Can you work these out from the model? Positions are in its coordinate system, mm. A direction names the side the tool comes from. Coordinates: 2 decimals unless noted, no trailing zeros. Return JSON: item names as keys, results as strings. Group by question number.
1) If we mould it in two halves opening along X, with no side actions, what happens to faces 1 (the face through (0, 0, 85)), 2 (the face through (-14.985, 0.66, 18.759)), 3 (the face through (-3, -10, 0)), 4 (the face through (-4.336, -19.524, 104.86))? For each: pulls with the +X half, pulls with the -X half, needs draft (parallel to the pull), parting line crosses it, or undercut.
2) If I drill on line 1 along Y through (x, z) = (0, 34.5); line 2 along Z through (x, y) = (11.5, 0); line 3 along Y through (x, z) = (0, 6), over which ranges is the centre line in solid material (lowest first)?
3) Which directions (+Z, -Z, +X, -X, +Y, -Y) give clear straight access to the entire face, cutting with the end or side of a thin tool? Please do faces 5 (the face through (0, 0, 95)), 6 (the face through (14.3, -14.3, 115)), 7 (the face through (0, 8.2, 13.797)).
4) For pin 1 Ø12 at (x, y) = (1.5, 4) entering from +Z; pin 2 Ø8 at (y, z) = (14, 68.5) entering from -X; pin 3 Ø0.7 at (x, z) = (8, 29.5) entering from +Y, each with a flat end and sliding along its axis, tell me the tip position at first contact or that it passes through.
```python
from build123d import *

# Parameters (mm, degrees)
F3_DEPTH = 35


with BuildPart() as f1:
    # F0 (on Front) → F1 (revolve)
    with BuildSketch(Plane.XZ):
        with BuildLine():
            Line((10, 0), (15, 0))
            Line((15, 0), (15, 37))
            add(Edge.make_bspline(
                [(15, 37), (19.0353800747, 58.2166660939), (33.9262575449, 86.7684902948), (28.5537857562, 105.9863269329), (21.6, 115)],
                knots=[0, 0, 0, 0, 0.5797552931, 1, 1, 1, 1], degree=3))
            Line((21.6, 115), (20, 115))
            Line((20, 115), (20, 95))
            Line((20, 95), (0, 95))
            Line((0, 95), (0, 85))
            Line((0, 85), (8, 85))
            Line((8, 85), (8, 13.7968156487))
            Line((8, 13.7968156487), (10, 13.7968156487))
            Line((10, 13.7968156487), (10, 0))
        make_face()
    revolve(axis=Axis((0, 0, 90), (0, 0, 1)))

    # F2 (on face) → F3 (cut)
    with BuildSketch(Plane(origin=(0, 0, 13.7968156487), x_dir=(1, 0, 0), z_dir=(0, 0, -1))):
        with BuildLine():
            Line((-7.5993420768, 2.5), (-9, 2.5))
            Line((-9, 2.5), (-9, -2.5))
            Line((-9, -2.5), (-7.5993420768, -2.5))
            ThreePointArc((-7.5993420768, -2.5), (-8, 0), (-7.5993420768, 2.5))
        make_face()
        with BuildLine():
            Line((9, 2.5), (7.5993420768, 2.5))
            ThreePointArc((7.5993420768, 2.5), (7.8992004853, 1.2659509046), (8, 0))
            ThreePointArc((8, 0), (7.8992004853, -1.2659509046), (7.5993420768, -2.5))
            Line((7.5993420768, -2.5), (9, -2.5))
            Line((9, -2.5), (9, 2.5))
        make_face()
    extrude(amount=-F3_DEPTH, mode=Mode.SUBTRACT)


solid = f1.part
```
Calculated:
{
 "1": {"face 1": "undercut", "face 2": "parting line crosses it", "face 3": "needs draft", "face 4": "undercut"},
 "2": {"line 1": "-15 to -8, 8 to 15", "line 2": "0 to 95", "line 3": "-15 to -10, 10 to 15"},
 "3": {"face 5": "+Z", "face 6": "+Z, +X, -X, +Y, -Y", "face 7": "-Z"},
 "4": {"pin 1": "z = 95", "pin 2": "x = -22.44", "pin 3": "y = 12.9"}
}
